Can you work these out from the model? Positions are in its coordinate system, mm. A direction names the side the tool comes from. Coordinates: 2 decimals unless noted, no trailing zeros. Order: outer loops, then holes, each group sorted by start corner. A loop starts at its lowest first (then second) coordinate and runs counter-clockwise, first axis right, second up. Notation, with made-up numbers: (69, 87.25) - (99, 87.25) arc R26 cw to (99, 125.25) - close; hole circle Ø2 at (-6.5, 40). An arc over 180 degrees is marked (long way). Return JSON: item names as keys, results as strings. Group by question number.
1) Imagine slicing it at A-A (z = -7.5). Write out the boundary of the cut face in (x, y).
2) If we mould it in two halves opening along X, with no side actions, what happens to faces 1 (the face through (44, 15, -6.1)), 2 (the face through (-80, 0, 0)), 3 (the face through (75, -25, 0))? For each: pulls with the +X half, pulls with the -X half, needs draft (parallel to the pull), parting line crosses it, or undercut.
3) For pin 1 Ø4 at (x, y) = (-41, -15) entering from +Z; pin 2 Ø5 at (x, y) = (-2.5, 23) entering from -Z, each with a flat end and sliding along its axis, tell me the tip position at first contact or that it passes through.
4) Imagine slicing it at B-B (x = -70). Write out the boundary of the cut face in (y, z), and give its area (3 significant figures).
5) If I drill on line 1 along Y through (x, z) = (50, 1.25); line 2 along Y through (x, z) = (-70, -0.75); line 3 along X through (y, z) = (10, 8.25), over which ranges is the centre line in solid material (lowest first)?
6) Imagine slicing it at D-D (z = 2.25). Write out the boundary of the cut face in (x, y), and give its area (3 significant figures).
7) Which directions (+Z, -Z, +X, -X, +Y, -Y) give clear straight access to the entire face, cutting with the end or side of a thin tool? Please do faces 4 (the face through (76.707, 8.41, -7.028)), 5 (the face through (44, 15, -4.5)), 6 (the face through (37.303, -9.736, -0.063)).
```python
from build123d import *

# Parameters (mm, degrees)
SKETCH1_W           = 160
SKETCH1_H           = 60
SKETCH1_R           = 4.25
SKETCH1_R_2         = 16
BOSS_EXTRUDE1_DEPTH = 9
CIRPATTERN2_COUNT   = 3
CHAMFER1_SIZE       = 10
SKETCH5_R           = 18.5
SKETCH5_R_2         = 16
CUT_EXTRUDE2_DEPTH  = 1.6
SKETCH4_R           = 28
CUT_EXTRUDE1_DEPTH  = 4


with BuildPart() as part:
    # Sketch1 → Boss-Extrude1 (new body, symmetric)
    with BuildSketch(Plane.XY):
        Rectangle(SKETCH1_W, SKETCH1_H)
        with Locations((-70, 18)):
            Circle(SKETCH1_R, mode=Mode.SUBTRACT)
        with Locations((-70, -18)):
            Circle(SKETCH1_R, mode=Mode.SUBTRACT)
        with Locations((50, 0)):
            Circle(SKETCH1_R_2, mode=Mode.SUBTRACT)
    extrude(amount=BOSS_EXTRUDE1_DEPTH, both=True)

    # Sketch3 → M5 Tapped Hole1 (revolve, cut)
    with BuildSketch(Plane(origin=(50, 22.5, 9), x_dir=(0, -1, 0), z_dir=(1, 0, 0))):
        Polygon((0, 0), (0, 11.2618073), (2.1, 10), (2.1, 0), align=None)
    m5_tapped_hole1 = revolve(axis=Axis((50, 22.5, 15.35), (0, 0, -1)), mode=Mode.SUBTRACT)

    # CirPattern2: M5 Tapped Hole1 ×3 about axis
    cirpattern2_axis = Axis((50, 0, 0), (0, 0, 1))
    for i in range(1, CIRPATTERN2_COUNT):
        add(m5_tapped_hole1.rotate(cirpattern2_axis, i * 360 / CIRPATTERN2_COUNT), mode=Mode.SUBTRACT)

    # Chamfer1
    chamfer1_edges = [part.edges().sort_by_distance(p)[0] for p in [
        (80, 30, 0),
        (80, -30, 0),
    ]]
    chamfer(chamfer1_edges, length=CHAMFER1_SIZE)

    # Sketch5 → Cut-Extrude2 (cut)
    with BuildSketch(Plane.XY.offset(4.5)):
        with Locations((50, 0)):
            Circle(SKETCH5_R)
        with Locations((50, 0)):
            Circle(SKETCH5_R_2, mode=Mode.SUBTRACT)
    cut_extrude2 = extrude(amount=CUT_EXTRUDE2_DEPTH, mode=Mode.SUBTRACT)

    # Mirror2: Cut-Extrude2 across plane
    add(cut_extrude2.mirror(Plane.XY), mode=Mode.SUBTRACT)

    # Sketch4 → Cut-Extrude1 (cut)
    with BuildSketch(Plane.XY.offset(9)):
        with BuildLine():
            ThreePointArc((-55.830052443, 30), (-60, 0), (-55.830052443, -30))
            Line((-55.830052443, -30), (70, -30))
            Line((70, -30), (80, -20))
            Line((80, -20), (80, 20))
            Line((80, 20), (70, 30))
            Line((70, 30), (-55.830052443, 30))
        make_face()
        with Locations((50, 0)):
            Circle(SKETCH4_R, mode=Mode.SUBTRACT)
    cut_extrude1 = extrude(amount=-CUT_EXTRUDE1_DEPTH, mode=Mode.SUBTRACT)

    # Mirror1: Cut-Extrude1 across plane
    add(cut_extrude1.mirror(Plane.XY), mode=Mode.SUBTRACT)


solid = part.part
```
Calculated:
{
 "1": {"outline": "(-80, -30) - (-55.83, -30) arc R110 cw to (-55.83, 30) - (-80, 30) - close; circle Ø56 at (50, 0); hole circle Ø8.5 at (-70, -18); hole circle Ø8.5 at (-70, 18); hole circle Ø32 at (50, 0)"},
 "2": {"face 1": "undercut", "face 2": "pulls with the -X half", "face 3": "pulls with the +X half"},
 "3": {"pin 1": "z = 5", "pin 2": "z = -5"},
 "4": {"outline": "(-30, -9) - (-22.25, -9) - (-22.25, 9) - (-30, 9) - close; (-13.75, -9) - (13.75, -9) - (13.75, 9) - (-13.75, 9) - close; (22.25, -9) - (30, -9) - (30, 9) - (22.25, 9) - close", "area": "774 mm2"},
 "5": {"line 1": "-30 to -16, 16 to 20.4, 24.6 to 30", "line 2": "-30 to -22.25, -13.75 to 13.75, 22.25 to 30", "line 3": "-80 to -59.54, 23.85 to 37.51, 62.49 to 76.15"},
 "6": {"outline": "(-80, -30) - (70, -30) - (80, -20) - (80, 20) - (70, 30) - (-80, 30) - close; hole circle Ø8.5 at (-70, -18); hole circle Ø8.5 at (-70, 18); hole circle Ø4.2 at (30.51, -11.25); hole circle Ø32 at (50, 0); hole circle Ø4.2 at (50, 22.5); hole circle Ø4.2 at (69.49, -11.25)", "area": "8,540 mm2"},
 "7": {"face 4": "-Z", "face 5": "none", "face 6": "+Z, -Z"}
}
